The model under review builds one solid part; all positions refer to its coordinate system, in mm. Face numbers are marked on the shaded views. A direction names the side the tool comes from. Coordinates: 2 decimals unless noted, no trailing zeros. Write each loop counter-clockwise with the first axis right and the second up, starting at its lowest first coordinate (ties: lowest second). Pieces come first, ordered by that corner, then holes. Notation, with made-up numbers: (63, -23.5) - (117, -23.5) arc R34 ccw to (117, 9.5) - close; hole circle Ø2 at (41, 57). An arc over 180 degrees is marked (long way). Put each result on its own line as item: value.
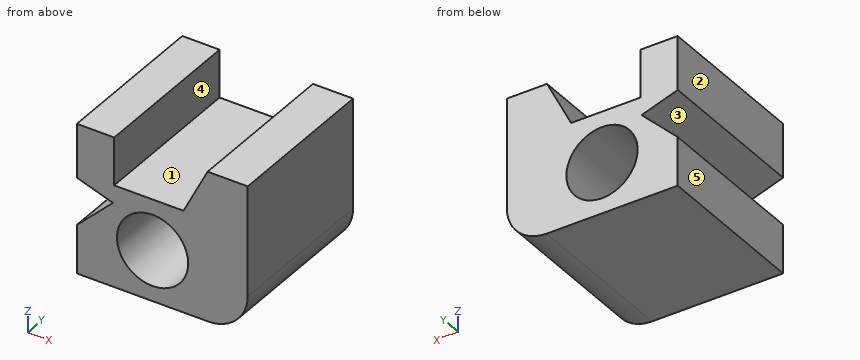
from build123d import *

# Parameters (mm, degrees)
F0_R     = 11.380259
F1_DEPTH = 50.8


with BuildPart() as f1:
    # F0 (on Front) → F1 (new body)
    with BuildSketch(Plane.XZ):
        with BuildLine():
            Line((-42.685506, 26.217468), (-54.612678, 26.217468))
            Line((-54.612678, 26.217468), (-54.612678, 8.996693))
            Line((-54.612678, 8.996693), (-43.042839, 5.175187))
            Line((-43.042839, 5.175187), (-54.612678, -6.061751))
            Line((-54.612678, -6.061751), (-54.612678, -21.593322))
            Line((-54.612678, -21.593322), (-12.7, -21.593322))
            ThreePointArc((-12.7, -21.593322), (-3.719744, -17.873578), (0, -8.893322))
            Line((0, -8.893322), (0, 26.217468))
            Line((0, 26.217468), (-12.834665, 26.217468))
            Line((-12.834665, 26.217468), (-20.538239, 10.913563))
            Line((-20.538239, 10.913563), (-42.685506, 10.913563))
            Line((-42.685506, 10.913563), (-42.685506, 26.217468))
        make_face()
        with Locations((-30.412134, -5.377338)):
            Circle(F0_R, mode=Mode.SUBTRACT)
    extrude(amount=F1_DEPTH)


solid = f1.part
1. Consider section A-A on z = 15.5. State the section outline as (x, y) points.
Determined:
outline: (-54.61, -50.8) - (-42.69, -50.8) - (-42.69, 0) - (-54.61, 0) - close; (-18.23, -50.8) - (0, -50.8) - (0, 0) - (-18.23, 0) - close
2. Consider section D-D on x = -15.5. State the section outline as (y, z) points.
Determined:
outline: (-50.8, -21.59) - (0, -21.59) - (0, 20.92) - (-50.8, 20.92) - close
3. The part is to be moulded in two halves that separate along Z. For the marked faces 1, 2 and 3, say which applies: +Z half, -Z half, draft (parallel to the pull), parting line (faces both ways), or undercut.
Determined:
face 1: +Z half
face 2: draft
face 3: undercut
4. For pin 1 Ø3 at (y, z) = (-19.5, -7) entering from +X; pin 2 Ø1 at (x, y) = (-19.5, -27) entering from +Z; pin 3 Ø6.5 at (x, y) = (-30, -28.5) entering from +Z, all flat-tipped, find the tip position at first contact; note any pin that passes through.
Determined:
pin 1: stops at x = 0
pin 2: stops at z = 13.97
pin 3: stops at z = 10.91
5. Machinability: for the marked faces 4 and 5, which of the approach directions +Z, -Z, +X, -X, +Y, -Y give a long, thin tool a straight path to every point of the face, cutting with its end or side? Answer none if there is none.
Determined:
face 4: +Z, +Y, -Y
face 5: +Z, -Z, -X, +Y, -Y
6. To check wall thickness, follow probe 1 along Z at (x, y) = (-48, -25); probe 2 along X at (y, z) = (-26.5, 3); probe 3 along Z at (x, y) = (-50, -44.5). State the ranges of each line that lie inside material, in increasing order.
Determined:
probe 1: z = -21.59 to 0.36, 6.81 to 26.22
probe 2: x = -45.28 to -38.11, -22.71 to 0
probe 3: z = -21.59 to -1.58, 7.47 to 26.22
7. Consider section C-C on y = -45. State the section outline as (x, z) points, plus the area to 3 significant figures.
Determined:
outline: (-54.61, -21.59) - (-12.7, -21.59) arc R12.7 ccw to (0, -8.89) - (0, 26.22) - (-12.83, 26.22) - (-20.54, 10.91) - (-42.69, 10.91) - (-42.69, 26.22) - (-54.61, 26.22) - (-54.61, 9) - (-43.04, 5.18) - (-54.61, -6.06) - close; hole circle Ø22.76 at (-30.41, -5.38)
area: 1,680 mm^2
8. Consider section B-B on x = -32.5. State the section outline as (y, z) points, plus the area to 3 significant figures.
Determined:
outline: (-50.8, -21.59) - (0, -21.59) - (0, -16.56) - (-50.8, -16.56) - close; (-50.8, 5.81) - (0, 5.81) - (0, 10.91) - (-50.8, 10.91) - close
area: 515 mm^2
